from build123d import *

# Parameters (mm, degrees)
SKETCH_R        = 20
SKETCH_R_2      = 16
PAD_DEPTH       = 11
SKETCH001_R     = 30
PAD001_DEPTH    = 3
SKETCH002_R     = 16
SKETCH002_R_2   = 14
PAD002_DEPTH    = 1
SKETCH003_R     = 14
POCKET_DEPTH    = 3.001
SKETCH004_R     = 16
PAD003_DEPTH    = 14
PAD004_DEPTH    = 2.5
SKETCH007_R     = 2.15
SKETCH007_R_2   = 2.65
POCKET001_DEPTH = 23.501
SKETCH008_R     = 2.15
POCKET002_DEPTH = 3.001
SKETCH009_R     = 4.75
POCKET003_DEPTH = 13.501
PAD005_DEPTH    = 7
SKETCH011_R     = 2.15
SKETCH011_R_2   = 2.65
POCKET004_DEPTH = 23.501
FILLET_R        = 1
CHAMFER_SIZE    = 0.7
FILLET001_R     = 1
POCKET005_DEPTH = 6


with BuildPart() as part:
    # Sketch → Pad (new body)
    with BuildSketch(Plane.XY):
        Circle(SKETCH_R)
        Circle(SKETCH_R_2, mode=Mode.SUBTRACT)
    extrude(amount=PAD_DEPTH)

    # Sketch001 (on Face4 of Pad) → Pad001 (join)
    with BuildSketch(Plane.XY.offset(11)):
        Circle(SKETCH001_R)
    extrude(amount=PAD001_DEPTH)

    # Sketch002 (on Face7 of Pad001) → Pad002 (join)
    with BuildSketch(Plane(origin=(0, 0, 11), x_dir=(1, 0, 0), z_dir=(0, 0, -1))):
        Circle(SKETCH002_R)
        Circle(SKETCH002_R_2, mode=Mode.SUBTRACT)
    extrude(amount=PAD002_DEPTH)

    # Sketch003 (on Face9 of Pad002) → Pocket (cut, through all)
    with BuildSketch(Plane(origin=(0, 0, 11), x_dir=(1, 0, 0), z_dir=(0, 0, -1))):
        Circle(SKETCH003_R)
    extrude(amount=-POCKET_DEPTH, mode=Mode.SUBTRACT)

    # Sketch004 (on Face6 of Pocket) → Pad003 (join)
    with BuildSketch(Plane(origin=(0, 0, 0), x_dir=(1, 0, 0), z_dir=(0, 0, -1))):
        with BuildLine():
            ThreePointArc((-8.717798, -18), (20, 0), (-8.717798, 18))
            Line((-30, 18), (-8.717798, 18))
            Line((-30, -18), (-30, 18))
            Line((-8.717798, -18), (-30, -18))
        make_face()
        Circle(SKETCH004_R, mode=Mode.SUBTRACT)
    extrude(amount=-PAD003_DEPTH)

    # Sketch005 (on Face9 of Pad003) → Pad004 (join)
    with BuildSketch(Plane(origin=(0, 0, 0), x_dir=(1, 0, 0), z_dir=(0, 0, -1))):
        with BuildLine():
            Line((-30, 18), (-13.5, 18))
            Line((-13.5, 18), (-13.5, 10.331989))
            ThreePointArc((-13.5, 10.331989), (-17, 0), (-13.5, -10.331989))
            Line((-13.5, -10.331989), (-13.5, -18))
            Line((-13.5, -18), (-30, -18))
            Line((-30, -18), (-30, 18))
        make_face()
    extrude(amount=PAD004_DEPTH)

    # Sketch007 → Pocket001 (cut, through all)
    with BuildSketch(Plane(origin=(0, 0, -9.5), x_dir=(1, 0, 0), z_dir=(0, 0, -1))):
        with Locations((-20, 13)):
            Circle(SKETCH007_R)
        with Locations((-20, -13)):
            Circle(SKETCH007_R_2)
    extrude(amount=-POCKET001_DEPTH, mode=Mode.SUBTRACT)

    # Sketch008 (on Face2 of Pocket001) → Pocket002 (cut, through all)
    with BuildSketch(Plane(origin=(0, 0, 11), x_dir=(1, 0, 0), z_dir=(0, 0, -1))):
        with Locations((25, 0)):
            Circle(SKETCH008_R)
        with Locations((-12.5, 21.650635)):
            Circle(SKETCH008_R)
        with Locations((-12.5, -21.650635)):
            Circle(SKETCH008_R)
    extrude(amount=-POCKET002_DEPTH, mode=Mode.SUBTRACT)

    # Sketch009 (on Face2 of Pocket002) → Pocket003 (cut, through all)
    with BuildSketch(Plane(origin=(0, 0, 11), x_dir=(1, 0, 0), z_dir=(0, 0, -1))):
        with Locations((-12.5, -21.650635)):
            Circle(SKETCH009_R)
        with Locations((-12.5, 21.650635)):
            Circle(SKETCH009_R)
    extrude(amount=POCKET003_DEPTH, mode=Mode.SUBTRACT)

    # Sketch010 (on Face30 of Pocket003) → Pad005 (join)
    with BuildSketch(Plane(origin=(0, 0, -2.5), x_dir=(1, 0, 0), z_dir=(0, 0, -1))):
        with BuildLine():
            ThreePointArc((-15, -13), (-23.605937, -9.536299), (-19.798889, -17.995954))
            Line((-19.798889, -17.995954), (-16.5, -17.995954))
            Line((-16.5, -17.995954), (-15, -16.495954))
            Line((-15, -13), (-15, -16.495954))
        make_face()
        with BuildLine():
            ThreePointArc((-20, 18), (-23.535534, 9.464466), (-15, 13))
            Line((-15, 13), (-15, 16.5))
            Line((-16.5, 18), (-15, 16.5))
            Line((-20, 18), (-16.5, 18))
        make_face()
    extrude(amount=PAD005_DEPTH)

    # Sketch011 (on Face49 of Pad005) → Pocket004 (cut, through all)
    with BuildSketch(Plane(origin=(0, 0, -9.5), x_dir=(1, 0, 0), z_dir=(0, 0, -1))):
        with Locations((-20, 13)):
            Circle(SKETCH011_R)
        with Locations((-20, -13)):
            Circle(SKETCH011_R_2)
    extrude(amount=-POCKET004_DEPTH, mode=Mode.SUBTRACT)

    # Fillet
    fillet_edges = [part.edges().sort_by_distance(p)[0] for p in [
        (-16.5, 17.995954, -6),
        (-15, 16.495954, -6),
        (-15, -16.5, -6),
        (-16.5, -18, -6),
    ]]
    fillet(fillet_edges, radius=FILLET_R)

    # Chamfer
    chamfer_edges = [part.edges().sort_by_distance(p)[0] for p in [
        (-16, 0, 0),
    ]]
    chamfer(chamfer_edges, length=CHAMFER_SIZE)

    # Fillet001
    fillet001_edges = [part.edges().sort_by_distance(p)[0] for p in [
        (-30, 18, 7),
        (-30, 18, -1.25),
        (-30, -18, -1.25),
        (-30, -18, 7),
    ]]
    fillet(fillet001_edges, radius=FILLET001_R)

    # Sketch012 (on Face50 of Fillet001) → Pocket005 (cut)
    with BuildSketch(Plane.XY.offset(14)):
        with BuildLine():
            ThreePointArc((-21.553244, 8.247376), (-15.062485, 12.212001), (-19.996782, 17.999999))
            Line((-19.996782, 17.999999), (-19.996782, 34.276657))
            Line((-19.996782, 34.276657), (-36.551773, 8.247376))
            Line((-21.553244, 8.247376), (-36.551773, 8.247376))
        make_face()
        with BuildLine():
            ThreePointArc((-20, -18), (-15, -13), (-20, -8))
            Line((-20, -8), (-40.401188, -8))
            Line((-20, -33.121502), (-40.401188, -8))
            Line((-20, -18), (-20, -33.121502))
        make_face()
    extrude(amount=-POCKET005_DEPTH, mode=Mode.SUBTRACT)


solid = part.part
Work out the finished part from the listing and answer in its coordinate system (mm). A direction names the side the tool comes from. Coordinates: 2 decimals unless noted, no trailing zeros. Loops run counter-clockwise (first coordinate to the right, second up) from the corner with the lowest first, then second, coordinate; pieces in that order, holes last. Notation, with made-up numbers: M -19,12.5 L -2,12.5 A11 cw -2,32.5 Z; hole C 37.25,27 d6. An arc over 180 degrees is marked long. Answer in a Markdown table with one row per item. Add a question column.
1. Flat-ended cylindrical pins translate along their axes: P1, Ø3.5, axis at y = 14.5, z = -4.5, coming from the +X side; P2, Ø2, axis at y = -14.5, z = -1.5, coming from the +X side; P3, Ø4, axis at x = -4, z = 2, coming from the +Y side. Find the tip coordinate at first contact, or state that the pin passes through.
2. A tool of negligible diameter and unlimited length cuts with its end or side. For faces 1 (the flat face through (-20, -20, 13)), 2 (the cylindrical face through (-15, -13, 11)), 3 (the cylindrical face through (-12.5, -16.9, 5.8)), 4 (the flat face through (-18, 17.996, -6)), 5 (the flat face through (-26, 8.247, 11)), from which of +Z, -Z, +X, -X, +Y, -Y can it reach the whole face along a straight path? Write none if from no direction.
3. Find section A-A, the plane x = 0. Write down the section's boundary in (y, z), then the cut area to 3 significant figures.
4. Consider L1, parallel to Y at x = -20, z = 0.5; L2, parallel to X at y = -13, z = -7.5; L3, parallel to X at y = 0, z = 5.5. Determine where each line is inside the solid, lowest interval first.
5. The mould has two halves that part along Y. Classify faces 6 (the flat face through (-22, -18, 3)), 7 (the flat face through (-19.997, 20, 12)), 8 (the cylindrical face through (-3.47, -15.62, 5.28)): pulls with the +Y half, pulls with the -Y half, needs draft (parallel to the pull), parting line crosses it, or undercut.
6. Find section D-D, the plane z = 12.25. Write down the section's boundary in (x, y).
7. Find section C-C, the plane z = 6.5. Write down the section's boundary in (x, y).
8. Find section B-B, the plane z = -6.5. Write down the section's boundary in (x, y).
Reported:
| question | item | result |
|---|---|---|
| 1 | P1 | stops at x = -15 |
| 1 | P2 | stops at x = -13.5 |
| 1 | P3 | stops at y = 19.9 |
| 2 | face 1 | +Z, -Z, -X, -Y |
| 2 | face 2 | +Z, -X |
| 2 | face 3 | -Z, -Y |
| 2 | face 4 | -Z, +X, -X, +Y |
| 2 | face 5 | +Z, -X, +Y |
| 3 | outline | M -30,11 L -20,11 L -20,0 L -16.7,0 L -16,0.7 L -16,10 L -14,10 L -14,14 L -30,14 Z; M 14,10 L 16,10 L 16,0.7 L 16.7,0 L 20,0 L 20,11 L 30,11 L 30,14 L 14,14 Z |
| 3 | area | 188 mm^2 |
| 4 | L1 | y = -18 to -15.15, -10.85 to 10.35, 15.65 to 18 |
| 4 | L2 | x = -25 to -22.15, -17.85 to -15 |
| 4 | L3 | x = -30 to -16, 16 to 20 |
| 5 | face 6 | pulls with the -Y half |
| 5 | face 7 | needs draft |
| 5 | face 8 | undercut |
| 6 | outline | M -30,-8 L -20,-8 A5 cw -20,-18 L -20,-22.36 A30 ccw long -20,22.36 L -20,18 A5 cw long -21.55,8.25 L -30,8.25 Z; hole C -12.5,-21.65 d4.3; hole C -12.5,21.65 d4.3; hole C 0,0 d28; hole C 25,0 d4.3 |
| 7 | outline | M -30,-17 A1 ccw -29,-18 L -15.54,-18 A4.75 cw -9.46,-18 L -8.72,-18 A20 ccw long -8.72,18 L -9.46,18 A4.75 cw -15.54,18 L -29,18 A1 ccw -30,17 Z; hole C -20,13 d5.3; hole C -20,-13 d4.3; hole C 0,0 d32 |
| 8 | outline | M -20,-18 L -16.91,-18 A1 ccw -16.21,-17.71 L -15.29,-16.79 A1 ccw -15,-16.09 L -15,-13 A5 ccw long Z; M -19.8,18 A5 ccw long -15,13 L -15,16.08 A1 ccw -15.29,16.79 L -16.21,17.7 A1 ccw -16.91,18 Z; hole C -20,13 d5.3; hole C -20,-13 d4.3 |
